from build123d import *

# Parameters (mm, degrees)
SKETCH1_R           = 2.25
BOSS_EXTRUDE1_DEPTH = 2
SKETCH2_W           = 35
SKETCH2_H           = 15
BOSS_EXTRUDE2_DEPTH = 31
CUT_EXTRUDE1_DEPTH  = 10
SKETCH4_R           = 2
CUT_EXTRUDE2_DEPTH  = 49.3741925
CHAMFER1_SIZE       = 3
SKETCH11_W          = 16
SKETCH11_H          = 12
CUT_EXTRUDE4_DEPTH  = 4
SKETCH13_W          = 3
SKETCH13_H          = 12
CUT_EXTRUDE5_DEPTH  = 2
BOSS_EXTRUDE7_DEPTH = 2
FILLET1_R           = 1
SKETCH15_R          = 0.5
CUT_EXTRUDE6_DEPTH  = 7
CUT_EXTRUDE7_START  = -2
SKETCH16_R          = 0.5
CUT_EXTRUDE7_DEPTH  = 18


with BuildPart() as part:
    # Sketch1 → Boss-Extrude1 (new body)
    with BuildSketch(Plane.XY):
        with BuildLine():
            Line((-18.9524457, 24.370059236), (23.0475543, -14.129940764))
            ThreePointArc((23.0475543, -14.129940764), (23.370059236, -21.5475543), (15.9524457, -21.870059236))
            Line((15.9524457, -21.870059236), (-26.0475543, 16.629940764))
            ThreePointArc((-26.0475543, 16.629940764), (-26.370059236, 24.0475543), (-18.9524457, 24.370059236))
        make_face()
        with Locations((-22.5, 20.5)):
            Circle(SKETCH1_R, mode=Mode.SUBTRACT)
        with Locations((19.5, -18)):
            Circle(SKETCH1_R, mode=Mode.SUBTRACT)
    extrude(amount=BOSS_EXTRUDE1_DEPTH)

    # Sketch2 → Boss-Extrude2 (add)
    with BuildSketch(Plane(origin=(0, 0, 2), x_dir=(-1, 0, 0), z_dir=(0, 0, -1))):
        with Locations((6.75, -8.75)):
            Rectangle(SKETCH2_W, SKETCH2_H)
    extrude(amount=BOSS_EXTRUDE2_DEPTH)

    # Sketch3 → Cut-Extrude1 (cut)
    with BuildSketch(Plane(origin=(0, 0, -29), x_dir=(-1, 0, 0), z_dir=(0, 0, -1))):
        Polygon((22.25, -13.25), (22.25, -6.25), (4.25, -6.25), (4.25, -13.25), (-10.75, -13.25), (-10.75, -16.25), (24.25, -16.25), (24.25, -13.25), align=None)
    extrude(amount=-CUT_EXTRUDE1_DEPTH, mode=Mode.SUBTRACT)

    # Sketch4 → Cut-Extrude2 (cut, through all)
    with BuildSketch(Plane(origin=(0, -1.25, 0), x_dir=(1, 0, 0), z_dir=(0, 1, 0))):
        with Locations(Location((-13.25, 26.3, 0), (0, 0, 270))):
            Circle(SKETCH4_R)
    extrude(amount=-CUT_EXTRUDE2_DEPTH, mode=Mode.SUBTRACT)

    # Chamfer1
    chamfer1_edges = [part.edges().sort_by_distance(p)[0] for p in [
        (10.75, -9.553591328, 0),
    ]]
    chamfer(chamfer1_edges, length=CHAMFER1_SIZE)

    # Sketch7 → Ø12.0mm Clearance Dowel Hole1 (revolve, cut)
    with BuildSketch(Plane(origin=(2.25, -16.25, -8.5), x_dir=(0, 0, -1), z_dir=(1, 0, 0))):
        Polygon((0, 0), (0, 15), (6.5, 15), (6.2, 14.7), (6.2, 0.2), (6.4, 0), align=None)
    revolve(axis=Axis((2.25, -22.6, -8.5), (0, 1, 0)), mode=Mode.SUBTRACT)

    # Sketch11 → Cut-Extrude4 (cut)
    with BuildSketch(Plane(origin=(0, 0, -29), x_dir=(-1, 0, 0), z_dir=(0, 0, -1))):
        with Locations((-2.75, -7.25)):
            Rectangle(SKETCH11_W, SKETCH11_H)
    extrude(amount=-CUT_EXTRUDE4_DEPTH, mode=Mode.SUBTRACT)

    # Sketch13 → Cut-Extrude5 (cut)
    with BuildSketch(Plane(origin=(0, 0, -29), x_dir=(-1, 0, 0), z_dir=(0, 0, -1))):
        with Locations((22.75, -7.25)):
            Rectangle(SKETCH13_W, SKETCH13_H)
    extrude(amount=-CUT_EXTRUDE5_DEPTH, mode=Mode.SUBTRACT)

    # Sketch9 → Boss-Extrude7 (add)
    with BuildSketch(Plane(origin=(0, 0, 2), x_dir=(-1, 0, 0), z_dir=(0, 0, -1))):
        Polygon((24.25, -1.25), (24.25, 14.982182656), (6.542164375, -1.25), align=None)
    extrude(amount=BOSS_EXTRUDE7_DEPTH)

    # Fillet1
    fillet1_edges = [part.edges().sort_by_distance(p)[0] for p in [
        (10.75, -1.25, -11.5),
        (3.25, -13.25, -25),
        (10.75, -7.25, -25),
        (2.75, -1.25, -25),
        (-23.25, -13.25, -27),
        (-24.25, -1.25, -13.5),
        (-24.25, -7.25, -27),
        (-22.75, -1.25, -27),
    ]]
    fillet(fillet1_edges, radius=FILLET1_R)

    # Sketch15 → Cut-Extrude6 (cut)
    with BuildSketch(Plane.XZ.offset(13.25)):
        with Locations((-4.25, -19)):
            Circle(SKETCH15_R)
        with Locations((-22.25, -19)):
            Circle(SKETCH15_R)
    extrude(amount=-CUT_EXTRUDE6_DEPTH, mode=Mode.SUBTRACT)

    # Sketch16 → Cut-Extrude7 (cut)
    with BuildSketch(Plane.ZY.offset(24.25).offset(CUT_EXTRUDE7_START)):
        with Locations((-19, -6.25)):
            Circle(SKETCH16_R)
    extrude(amount=-CUT_EXTRUDE7_DEPTH, mode=Mode.SUBTRACT)


solid = part.part
Design review of the part built by this model. Coordinates are the model's own, in mm. A direction names the side the tool comes from. Round coordinates to 2 decimals unless told otherwise and drop trailing zeros. Write each loop counter-clockwise with the first axis right and the second up, starting at its lowest first coordinate (ties: lowest second). Pieces come first, ordered by that corner, then holes. Notation, with made-up numbers: (83.25, -12) -> (109.25, -12) arc R12 ccw to (109.25, -1) -> close; hole circle Ø2 at (47, 4.25). An arc over 180 degrees is marked (long way). One line per item, written item: value. Start each with the question number.
Q1. To check wall thickness, follow probe 1 along Z at (x, y) = (-13, -6); probe 2 along X at (y, z) = (-4.5, -18); probe 3 along Y at (x, z) = (-14, -3). State the ranges of each line that lie inside material, in increasing order.
Q2. Add section D-D (y = -4). Give the boundary of the cut face in (x, z).
Q3. Tool access review of faces 1 (the face through (-23, -13.25, -23)), 2 (the face through (12.27, -9.46, -1.48)), 3 (the face through (-24.25, -8, -9)), 4 (the face through (-22.25, -10, -23)), 5 (the face through (-22, -6, -27)): name each direction out of +Z, -Z, +X, -X, +Y, -Y from which nothing blocks a thin tool from reaching the whole face with its end or side.
Q4. Insertion check: P1, Ø12, axis at x = 12.5, z = -19, coming from the +Y side; P2, Ø6, axis at x = -5, y = -1, coming from the -Z side; P3, Ø3, axis at x = 0.5, y = 6.5, coming from the -Z side; P4, Ø16.5, axis at x = 20, y = -10, coming from the -Z side. Each pin has a flat end and moves straight along its axis. Give the tip position at first contact, or say it passes through.
Q5. Add section B-B (y = 20.5). Give the boundary of the cut face in (x, z), then the cut area to 3 significant figures.
Q6. Add section C-C (z = -21). Give the boundary of the cut face in (x, y), then the cut area to 3 significant figures.
Q7. Add section A-A (x = 18). Give the boundary of the cut face in (y, z).
Q8. The part is to be moulded in two halves that separate along X. For faces 6 (the face through (-10, -12, -19)), 7 (the face through (12.93, -19.1, 0.99)), 8 (the face through (3, -13.25, -22)), say which applies: pulls with the +X half, pulls with the -X half, needs draft (parallel to the pull), parting line crosses it, or undercut.
Response:
1. probe 1: z = -29 to -28.28, -24.32 to -19.43, -18.57 to 2
1. probe 2: x = -24.25 to 10.75
1. probe 3: y = -16.25 to -1.25
2. outline: (-24.25, -26) arc R1 ccw to (-23.25, -27) -> (-21.25, -27) -> (-21.25, -29) -> (-5.25, -29) -> (-5.25, -25) -> (9.75, -25) arc R1 ccw to (10.75, -24) -> (10.75, -3) -> (12, -1.75) -> (12, 2) -> (-24.25, 2) -> close; hole circle Ø4 at (-13.25, -26.3); hole circle Ø12.4 at (2.25, -8.5)
3. face 1: -Z, +X, -X, -Y
3. face 2: -Z, +X, +Y, -Y
3. face 3: +Z, -Z, -X, -Y
3. face 4: -Z, -Y
3. face 5: -Z, -X, +Y, -Y
4. P1: stops at y = -1.25
4. P2: stops at z = -29
4. P3: stops at z = 0
4. P4: stops at z = -2
5. outline: (-27.75, 0) -> (-24.75, 0) -> (-24.75, 2) -> (-27.75, 2) -> close; (-20.25, 0) -> (-14.73, 0) -> (-14.73, 2) -> (-20.25, 2) -> close
5. area: 17.0 mm^2
6. outline: (-24.25, -13.25) -> (-22.25, -13.25) -> (-22.25, -6.25) -> (-4.25, -6.25) -> (-4.25, -13.25) -> (10.75, -13.25) -> (10.75, -2.25) arc R1 ccw to (9.75, -1.25) -> (-23.25, -1.25) arc R1 ccw to (-24.25, -2.25) -> close
6. area: 294 mm^2
7. outline: (-23.03, 0) -> (-19.68, 0) -> (-19.68, 2) -> (-23.03, 2) -> close; (-16.32, 0) -> (-9.5, 0) -> (-9.5, 2) -> (-16.32, 2) -> close
8. face 6: undercut
8. face 7: pulls with the -X half
8. face 8: needs draft
